Geometry: final body of the model. Coordinates: model frame, mm. Face numbers are marked on the shaded views. A direction names the side the tool comes from. Round coordinates to 2 decimals unless told otherwise and drop trailing zeros. Loops run counter-clockwise (first coordinate to the right, second up) from the corner with the lowest first, then second, coordinate; pieces in that order, holes last. Notation, with made-up numbers: M -21,-13 L -6,-13 A28 cw -6,17 Z; hole C -30.75,-20.5 d6. An arc over 180 degrees is marked long. Write each question's results on one line, items separated by ' | '.
```python
from build123d import *

# Parameters (mm, degrees)
F0_W           = 228.6
F0_H           = 50.8
F1_DEPTH       = 50.8
F3_D           = 13.4874
F3_CBORE_D     = 20.6375
F3_CBORE_DEPTH = 17.78
F5_D           = 13.4874
F5_DEPTH       = 25.4
F5_CBORE_D     = 20.6375
F5_CBORE_DEPTH = 17.78


with BuildPart() as f1:
    # F0 (on Front) → F1 (new body)
    with BuildSketch(Plane.XZ):
        Rectangle(F0_W, F0_H)
    extrude(amount=F1_DEPTH)

    # F3 (through all)
    with Locations(Plane.XZ.offset(50.8)):
        with Locations((-88.9, 0), (0, 0), (88.9, 0)):
            CounterBoreHole(F3_D / 2, F3_CBORE_D / 2, F3_CBORE_DEPTH)

    # F5
    with Locations(Plane(origin=(0, 0, 0), x_dir=(1, 0, 0), z_dir=(0, 1, 0))):
        with Locations((88.9, 0), (0, 0), (-88.9, 0)):
            CounterBoreHole(F5_D / 2, F5_CBORE_D / 2, F5_CBORE_DEPTH, depth=F5_DEPTH)


solid = f1.part
```
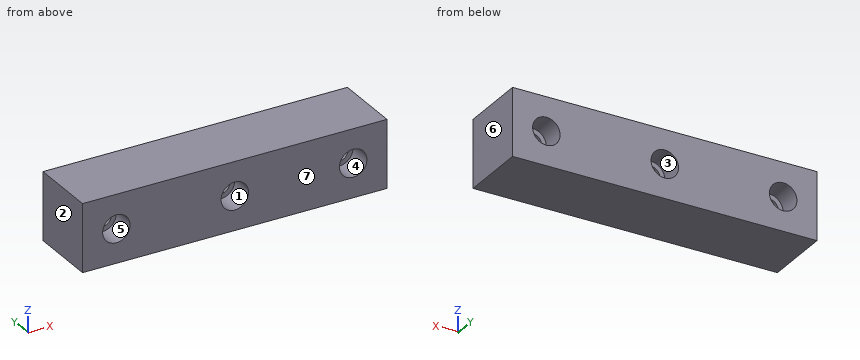
1. Draft query along X for the marked faces 4, 5, 6 and 7. Return one class per face: pulls with the +X half, pulls with the -X half, needs draft (parallel to the pull), parting line crosses it, or undercut.
Answer key:
face 4: undercut | face 5: undercut | face 6: pulls with the +X half | face 7: needs draft
2. Access query for the marked faces 1, 2 and 3. Directions: +Z, -Z, +X, -X, +Y, -Y. A direction counts if a zero-diameter tool reaches every point of the face in a straight line with its end or side. Return the directions, or none.
Answer key:
face 1: -Y | face 2: +Z, -Z, -X, +Y, -Y | face 3: +Y
3. Section C-C (z = 0). Count the separate pieces of the cut face and the enclosed holes in it, then the cut area to 3 significant figures.
Answer key:
separate pieces: 4 | enclosed holes: 0 | area: 8,790 mm²
4. Pin query (flat end, axial travel): P1, Ø11, axis at x = 88.9, z = 0, coming from the -Y side; P2, Ø16.5, axis at x = 0, z = 0, coming from the -Y side; P3, Ø6, axis at x = 3.5, z = 3.5, coming from the +Y side. Return the tip coordinate at first contact, or that it passes through.
Answer key:
P1: passes through | P2: stops at y = -33.02 | P3: stops at y = -17.78
5. Section A-A (x = 0). Output: boundary loops of the cut face in (y, z), then the cut area to 3 significant figures.
Answer key:
outline: M -50.8,-25.4 L 0,-25.4 L 0,-10.32 L -17.78,-10.32 L -17.78,-6.74 L -33.02,-6.74 L -33.02,-10.32 L -50.8,-10.32 Z; M -50.8,10.32 L -33.02,10.32 L -33.02,6.74 L -17.78,6.74 L -17.78,10.32 L 0,10.32 L 0,25.4 L -50.8,25.4 Z | area: 1,640 mm²
6. Ray query, probe 1 along X at (y, z) = (-38, -7); probe 2 along Z at (x, y) = (-88.9, -43); probe 3 along X at (y, z) = (-19.5, 5). Return the intervals inside material, ascending.
Answer key:
probe 1: x = -114.3 to -96.48, -81.32 to -7.58, 7.58 to 81.32, 96.48 to 114.3 | probe 2: z = -25.4 to -10.32, 10.32 to 25.4 | probe 3: x = -114.3 to -93.43, -84.37 to -4.53, 4.53 to 84.37, 93.43 to 114.3
7. Section B-B (y = -43.5). Output: boundary loops of the cut face in (x, z).
Answer key:
outline: M -114.3,-25.4 L 114.3,-25.4 L 114.3,25.4 L -114.3,25.4 Z; hole C -88.9,0 d20.64; hole C 0,0 d20.64; hole C 88.9,0 d20.64
